For this review, take the finished solid that the model builds, in its own axes (mm). Coordinates: 2 decimals unless noted, no trailing zeros. Write each loop counter-clockwise with the first axis right and the second up, starting at its lowest first coordinate (ties: lowest second). Pieces come first, ordered by that corner, then holes.
Autodesk Inventor part; units mm, degrees
ref_plane "YZ Plane" through (0, 0, 0) normal (1, 0, 0) x (0, 1, 0)
ref_plane "XZ Plane" through (0, 0, 0) normal (0, 1, 0) x (-1, 0, 0)
ref_plane "XY Plane" through (0, 0, 0) normal (0, 0, 1) x (1, 0, 0)
sketch "Sketch5" plane through (0, 0, 0) normal (0, 1, 0) x (-1, 0, 0)
  line L0 (-22.9, -32.9) -> (22.9, 32.9) construction
  line L1 (22.9, -32.9) -> (-22.9, 32.9) construction
  circle A0 centre (22.9, 32.9) radius 1.5
  circle A1 centre (22.9, -32.9) radius 1.5
  circle A2 centre (-22.9, 32.9) radius 1.5
  circle A3 centre (-22.9, -32.9) radius 1.5
  point P0 (0, 0)
  dimension "d6" = 45.8
  dimension "d7" = 65.8
  dimension "d8" = 3
  dimension "d9" = 3
  dimension "d10" = 3
  dimension "d11" = 3
sketch "Sketch8" plane through (0, 0, 0) normal (0, 1, 0) x (-1, 0, 0)
  line L0 (28.9, -23.5) -> (-28.9, 23.5) construction
  line L1 (-28.9, -23.5) -> (28.9, 23.5) construction
  circle A0 centre (28.9, 23.5) radius 1.5
  circle A1 centre (28.9, -23.5) radius 1.5
  circle A2 centre (-28.9, 23.5) radius 1.5
  circle A3 centre (-28.9, -23.5) radius 1.5
  point P0 (0, 0)
  dimension "d24" = 57.8
  dimension "d25" = 47
  dimension "d26" = 3
  dimension "d27" = 3
  dimension "d28" = 3
  dimension "d29" = 3
sketch "Sketch10" plane through (0, 0, 0) normal (0, 1, 0) x (-1, 0, 0)
  line L0 (-24.4, -34.4) -> (24.4, -34.4)
  line L1 (24.4, -34.4) -> (24.4, 34.4)
  line L2 (24.4, 34.4) -> (-24.4, 34.4)
  line L3 (-24.4, 34.4) -> (-24.4, -34.4)
  line L4 (-24.4, -34.4) -> (24.4, 34.4) construction
  line L5 (24.4, -34.4) -> (-24.4, 34.4) construction
  line L6 (-30.4, -25) -> (30.4, -25)
  line L7 (30.4, -25) -> (30.4, 25)
  line L8 (30.4, 25) -> (-30.4, 25)
  line L9 (-30.4, 25) -> (-30.4, -25)
  line L10 (-30.4, -25) -> (30.4, 25) construction
  line L11 (30.4, -25) -> (-30.4, 25) construction
  circle A0 centre (28.8992, 23.4996) radius 3
  circle A1 centre (22.8996, 32.8995) radius 3
  circle A2 centre (28.8992, -23.4965) radius 3
  circle A3 centre (22.8996, -32.9046) radius 3
  circle A4 centre (-28.9017, -23.4965) radius 3
  circle A5 centre (-22.8972, -32.9046) radius 3
  circle A6 centre (-28.9017, 23.4996) radius 3
  circle A7 centre (-22.8972, 32.8995) radius 3
  point P0 (0, 0)
  point P1 (24.4, 25)
  point P2 (24.4, 30.3016)
  point P3 (20.3018, 34.4)
  point P4 (-20.2994, 34.4)
  point P5 (-24.4, 30.303)
  point P6 (-24.4, 25)
  point P7 (-26.3038, 25)
  point P8 (-30.4, 20.9006)
  point P9 (-30.4, -20.8974)
  point P10 (-26.3056, -25)
  point P11 (-24.4, -25)
  point P12 (-24.4, -30.3081)
  point P13 (-20.2965, -34.4)
  point P14 (20.2989, -34.4)
  point P15 (24.4, -30.3067)
  point P16 (24.4, -25)
  point P17 (26.3031, -25)
  point P18 (30.4, -20.8989)
  point P19 (30.4, 20.902)
  point P20 (26.3013, 25)
  dimension "d46" = 48.8
  dimension "d47" = 68.8
  dimension "d48" = 60.8
  dimension "d49" = 50
  dimension "d50" = 6
  dimension "d51" = 6
  dimension "d52" = 6
  dimension "d53" = 6
  dimension "d54" = 6
  dimension "d55" = 6
  dimension "d56" = 6
  dimension "d57" = 6
extrude "Extrusion3" add sketch "Sketch10" along normal blind 2
extrude "Extrusion4" cut sketch "Sketch5" along normal blind 2
extrude "Extrusion5" cut sketch "Sketch8" along normal blind 2
sketch "Sketch11" plane through (0, 2, 0) normal (0, 1, 0) x (1, 0, 0)
  circle A0 centre (0, 0) radius 20
  dimension "d64" = 40
extrude "Extrusion6" cut sketch "Sketch11" against normal blind 2
properties part number "PCB Bracket 2"
Q1. Add section B-B (y = 1.25). Give the number of separate pieces and of enclosed holes in the cut face, then the cut area to 3 significant figures.
Ans:
separate pieces: 1
enclosed holes: 9
area: 2,730 mm2
Q2. For probe 1 along Z at (x, y) = (22.9, 0.8); probe 2 along Z at (x, y) = (28.9, 0.55); probe 3 along Z at (x, y) = (0, 0.8), list the stretches that pass through material, from the lowest coordinate up.
Ans:
probe 1: z = -35.9 to -34.4, -31.4 to 31.4, 34.4 to 35.9
probe 2: z = -26.5 to -25, -22 to 22, 25 to 26.5
probe 3: z = -34.4 to -20, 20 to 34.4
Q3. Add section A-A (z = 32.9). State the section outline as (x, y) points, then the cut area to 3 significant figures.
Ans:
outline: (-25.9, 0) - (-24.4, 0) - (-24.4, 2) - (-25.9, 2) - close; (-21.4, 0) - (21.4, 0) - (21.4, 2) - (-21.4, 2) - close; (24.4, 0) - (25.9, 0) - (25.9, 2) - (24.4, 2) - close
area: 91.6 mm2
Q4. Add section C-C (x = 0). State the section outline as (y, z) points.
Ans:
outline: (0, -34.4) - (2, -34.4) - (2, -20) - (0, -20) - close; (0, 20) - (2, 20) - (2, 34.4) - (0, 34.4) - close
Q5. Add section D-D (x = 22.9). State the section outline as (y, z) points.
Ans:
outline: (0, -35.9) - (2, -35.9) - (2, -34.4) - (0, -34.4) - close; (0, -31.4) - (2, -31.4) - (2, 31.4) - (0, 31.4) - close; (0, 34.4) - (2, 34.4) - (2, 35.9) - (0, 35.9) - close
Q6. Clearance check with flat-ended pins moving along their axes: pin 1 Ø3.5 at (x, z) = (-22.9, 32.9) entering from +Y; pin 2 Ø2.5 at (x, z) = (22.9, -32.9) entering from -Y; pin 3 Ø1 at (x, y) = (-25, 1.5) entering from +Z; pin 4 Ø0.6 at (y, z) = (1, -26.5) entering from -X. State where each tip first meets the part, or that it passes through.
Ans:
pin 1: stops at y = 2
pin 2: passes through
pin 3: stops at z = 35.44
pin 4: stops at x = -30.2
